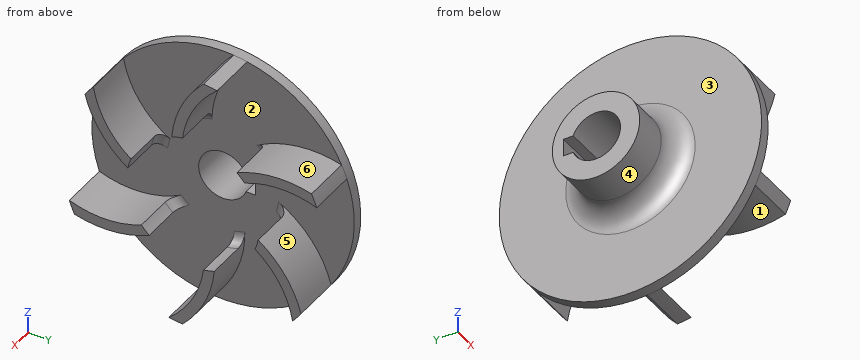
```python
from build123d import *
from build123d.topology import SkipClean

# Parameters (mm, degrees)
FILLET1_R                = 6
CUT_EXTRUDE1_DEPTH       = 20
BOSS_EXTRUDE1_DEPTH      = 14
FILLET2_R                = 3
CIRPATTERN1_COUNT        = 6
FILLET2_OF_CIRPATTERN1_R = 3


with BuildPart() as part:
    # Sketch1 → Revolve1 (revolve)
    with BuildSketch(Plane.XY, mode=Mode.PRIVATE) as revolve1_sk:
        Polygon((0, 7), (0, 12.5), (16, 12.5), (16, 37.5), (19, 37.5), (19, 7), align=None)
    revolve(revolve1_sk.sketch.rotate(Axis((-91.900691054, 0, 0), (1, 0, 0)), 90), axis=Axis((-91.900691054, 0, 0), (1, 0, 0)))  # turned: the seam where the file's is

    # Fillet1
    fillet1_edges = [part.edges().sort_by_distance(p)[0] for p in [
        (16, 0, -12.5),
    ]]
    fillet(fillet1_edges, radius=FILLET1_R)

    # Sketch2 → Cut-Extrude1 (cut, through all)
    with BuildSketch(Plane(origin=(19, 0, 0), x_dir=(0, 0, -1), z_dir=(1, 0, 0))):
        with BuildLine():
            Line((-2.5, 6.538348415), (-2.5, 9.3))
            Line((-2.5, 9.3), (2.5, 9.3))
            Line((2.5, 9.3), (2.5, 6.538348415))
            ThreePointArc((2.5, 6.538348415), (0, -7), (-2.5, 6.538348415))
        make_face()
    extrude(amount=-CUT_EXTRUDE1_DEPTH, mode=Mode.SUBTRACT)

    # Sketch3 → Boss-Extrude1 (add)
    with BuildSketch(Plane(origin=(19, 0, 0), x_dir=(0, 0, -1), z_dir=(1, 0, 0))):
        with BuildLine():
            ThreePointArc((-36.861475704, 6.890690018), (-28.755483578, 0.217996332), (-18.761663039, -3))
            ThreePointArc((-18.761663039, -3), (-18.443627284, -4.564275696), (-17.995407864, -6.09633462))
            ThreePointArc((-17.995407864, -6.09633462), (-28.49792429, -3.274961963), (-37.379807383, 3))
            ThreePointArc((-37.379807383, 3), (-37.171580486, 4.952131277), (-36.861475704, 6.890690018))
        make_face()
    boss_extrude1 = extrude(amount=BOSS_EXTRUDE1_DEPTH)

    # Fillet2
    fillet2_edges = [part.edges().sort_by_distance(p)[0] for p in [
        (19, -4.564275696, 18.443627284),
    ]]
    fillet(fillet2_edges, radius=FILLET2_R)

    # CirPattern1: Boss-Extrude1 ×6 about axis
    with SkipClean():  # keep this step's faces unmerged: merging them makes the solid invalid here
        cirpattern1_axis = Axis((0, 0, 0), (1, 0, 0))
        for i in range(1, CIRPATTERN1_COUNT):
            add(boss_extrude1.rotate(cirpattern1_axis, i * 360 / CIRPATTERN1_COUNT))

    # Fillet2 of CirPattern1
    fillet2_of_cirpattern1_edges = [part.edges().sort_by_distance(p)[0] for p in [
        (19, -18.254787613, 5.269034939),
        (19, -13.690511918, -13.174592344),
        (19, 4.564275696, -18.443627284),
        (19, 18.254787613, -5.269034939),
        (19, 13.690511918, 13.174592344),
    ]]
    fillet(fillet2_of_cirpattern1_edges, radius=FILLET2_OF_CIRPATTERN1_R)


solid = part.part
```
The model under review builds one solid part; all positions refer to its coordinate system, in mm. Face numbers are marked on the shaded views. A direction names the side the tool comes from. Coordinates: 2 decimals unless noted, no trailing zeros. Write each loop counter-clockwise with the first axis right and the second up, starting at its lowest first coordinate (ties: lowest second). Pieces come first, ordered by that corner, then holes. Notation, with made-up numbers: (53, -13.75) - (106, -13.75) arc R22 ccw to (106, 11.25) - close; hole circle Ø10 at (-20, 74.25). An arc over 180 degrees is marked (long way). Write item = value, one per line.
(1) For line 1 (Y direction, x = 8.75, z = 0); line 2 (X direction, y = -19.5, z = 10); line 3 (Y direction, x = 15, z = 3.5), list the stretches that pass through material, from the lowest coordinate up. Write a range as [from, to].
Result sheet:
line_1 = [-12.5, -7], [9.3, 12.5]
line_2 = [16, 19]
line_3 = [-14.77, -6.06], [6.06, 14.77]
(2) Consider section C-C, the plane y = -25. Give the boundary of the cut face in (x, z).
Result sheet:
outline = (16, -27.95) - (19, -27.95) - (19, -17.19) - (33, -17.19) - (33, -14.19) - (19, -14.19) - (19, 9.66) - (33, 9.66) - (33, 14.91) - (19, 14.91) - (19, 27.95) - (16, 27.95) - close
(3) For P1, Ø1.4, axis at x = 12, y = 8, coming from the -Z side; P2, Ø12, axis at x = 18, y = -26, coming from the -Z side; P3, Ø1, axis at x = 18, y = -22.5, coming from the -Z side; P4, Ø12, axis at y = -2.5, z = -22.5, coming from the +X side, all flat-tipped, find the tip position at first contact; note any pin that passes through.
Result sheet:
P1 = -10.67
P2 = -31.72
P3 = -30.37
P4 = 33
(4) Machinability: for the marked faces 4, 5 and 6, which of the approach directions +Z, -Z, +X, -X, +Y, -Y give a long, thin tool a straight path to every point of the face, cutting with its end or side? Answer none if there is none.
Result sheet:
face_4 = -X
face_5 = +X, +Y
face_6 = +Z, +X
(5) Consider section B-B, the plane x = 8.5. Give the boundary of the cut face in (y, z), then the cut area to 3 significant figures.
Result sheet:
outline = circle Ø25 at (0, 0); hole (6.54, -2.5) - (9.3, -2.5) - (9.3, 2.5) - (6.54, 2.5) arc R7 ccw (long way) to start
area = 325 mm^2
(6) Consider section D-D, the plane y = 0. Give the boundary of the cut face in (x, z), then the cut area to 3 significant figures.
Result sheet:
outline = (0, -12.5) - (10, -12.5) arc R6 cw to (16, -18.5) - (16, -37.5) - (19, -37.5) - (19, -33.94) - (33, -33.94) - (33, -28.35) - (19, -28.35) - (19, -7) - (0, -7) - close; (0, 7) - (19, 7) - (19, 28.35) - (33, 28.35) - (33, 33.94) - (19, 33.94) - (19, 37.5) - (16, 37.5) - (16, 18.5) arc R6 cw to (10, 12.5) - (0, 12.5) - close
area = 531 mm^2
(7) Mouldability with a two-part tool opening along Z and no side actions: class the marked faces 1, 2 and 3 as pulls with the +Z half, pulls with the -Z half, needs draft (parallel to the pull), parting line crosses it, or undercut.
Result sheet:
face_1 = pulls with the -Z half
face_2 = undercut
face_3 = needs draft
(8) Consider section A-A, the plane z = 0. Give the boundary of the cut face in (x, y), then the cut area to 3 significant figures.
Result sheet:
outline = (0, -12.5) - (10, -12.5) arc R6 cw to (16, -18.5) - (16, -37.5) - (19, -37.5) - (19, -7) - (0, -7) - close; (0, 9.3) - (19, 9.3) - (19, 37.5) - (16, 37.5) - (16, 18.5) arc R6 cw to (10, 12.5) - (0, 12.5) - close
area = 331 mm^2
